```python
from build123d import *

# Parameters (mm, degrees)
EXTRUDE_1_DEPTH           = 290
HOLE_WIZARD_5_0_5_1_D     = 5
HOLE_WIZARD_5_0_5_2_D     = 5
HOLE_WIZARD_5_0_5_2_DEPTH = 20
HOLE_WIZARD_5_0_5_2_TIP   = 1.502151548


with BuildPart() as part:
    # Sketch1 → 凸台-拉伸1 (new body)
    with BuildSketch(Plane.XY):
        Polygon((-6.5, 45), (-3.2, 45), (-3.2, 43.2), (-5.1, 43.2), (-5.1, 37.2), (5.1, 37.2), (5.1, 43.2), (3.2, 43.2), (3.2, 45), (6.5, 45), (7.5, 45), (7.5, 44), (7.5, 18.2), (5, 18.2), (5, 20.2), (-0.5, 20.2), (-0.5, 18.2), (-3, 18.2), (-3, 11.8), (-0.5, 11.8), (-0.5, 9.8), (5, 9.8), (5, 11.8), (7.5, 11.8), (7.5, -11.8), (5, -11.8), (5, -9.8), (-0.5, -9.8), (-0.5, -11.8), (-3, -11.8), (-3, -18.2), (-0.5, -18.2), (-0.5, -20.2), (5, -20.2), (5, -18.2), (7.5, -18.2), (7.5, -44), (7.5, -45), (6.5, -45), (3.2, -45), (3.2, -43.2), (5.1, -43.2), (5.1, -37.2), (-5.1, -37.2), (-5.1, -43.2), (-3.2, -43.2), (-3.2, -45), (-6.496721962, -45), (-7.5, -45), (-7.5, -44), (-7.5, -33.2), (-5, -33.2), (-5, -35.2), (0.5, -35.2), (0.5, -33.2), (3, -33.2), (3, -26.8), (0.5, -26.8), (0.5, -24.8), (-5, -24.8), (-5, -26.8), (-7.5, -26.8), (-7.5, -3.2), (-5, -3.2), (-5, -5.2), (0.5, -5.2), (0.5, -3.2), (3, -3.2), (3, 3.2), (0.5, 3.2), (0.5, 5.2), (-5, 5.2), (-5, 3.2), (-7.5, 3.2), (-7.5, 26.8), (-5, 26.8), (-5, 24.8), (0.5, 24.8), (0.5, 26.8), (3, 26.8), (3, 33.2), (0.5, 33.2), (0.5, 35.2), (-5, 35.2), (-5, 33.2), (-7.5, 33.2), (-7.5, 44), (-7.5, 45), align=None)
    extrude(amount=EXTRUDE_1_DEPTH)

    # Ø5.0 (5) 直径孔1 (through all)
    with Locations(Plane(origin=(7.5, 0, 0), x_dir=(0, 0, -1), z_dir=(1, 0, 0))):
        with Locations((-268, 30)):
            Hole(HOLE_WIZARD_5_0_5_1_D / 2)

    # Ø5.0 (5) 直径孔2
    with Locations(Plane(origin=(7.5, 0, 0), x_dir=(0, 0, -1), z_dir=(1, 0, 0))):
        with Locations((-217, 30.986103622), (-181, 30.986103622), (-109, 30.986103622), (-73, 30.986103622), (-22, 30.986103622), (-268, 0), (-217, -30), (-181, -30), (-163, 0), (-127, 0), (-109, -30), (-73, -30), (-22, 0)):
            Hole(HOLE_WIZARD_5_0_5_2_D / 2, depth=HOLE_WIZARD_5_0_5_2_DEPTH)
            with Locations((0, 0, -(HOLE_WIZARD_5_0_5_2_DEPTH + HOLE_WIZARD_5_0_5_2_TIP / 2))):  # 118° drill point
                Cone(0, HOLE_WIZARD_5_0_5_2_D / 2, HOLE_WIZARD_5_0_5_2_TIP, mode=Mode.SUBTRACT)


solid = part.part
```
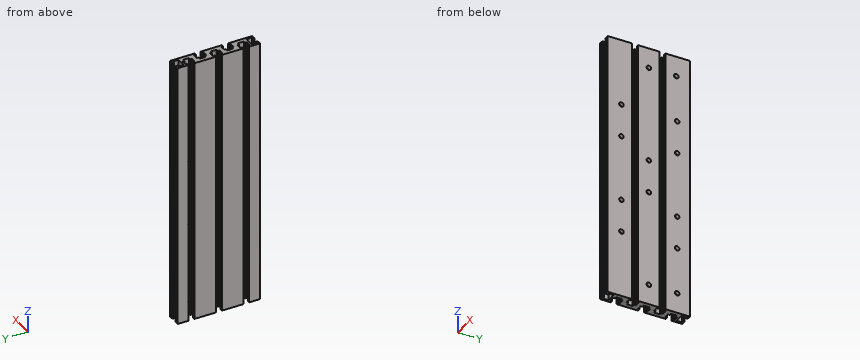
Could you check a few things on this model? Use its own coordinates, in mm. Round coordinates to 2 decimals unless told otherwise and drop trailing zeros. Order: outer loops, then holes, each group sorted by start corner. A loop starts at its lowest first (then second) coordinate and runs counter-clockwise, first axis right, second up. Notation, with made-up numbers: (30.25, -31) -> (63.25, -31) arc R16 cw to (63.25, -20) -> close; hole circle Ø7 at (58, 68.25). An arc over 180 degrees is marked (long way). One line per question, with ' | ' between items.
Q1. If we section it at C-C on y = -14.5: Write out the boundary of the cut face in (x, z).
Computed values:
outline: (-7.5, 0) -> (-3, 0) -> (-3, 290) -> (-7.5, 290) -> close
Q2. If I drill on line 1 (Y direction, x = -2.5, z = 183); line 2 (Y direction, x = 1.75, z = 107); line 3 (Y direction, x = -5.25, z = 125.5), over which ranges is the centre line in solid material (lowest first)? Write a range as from..to.
Computed values:
line 1: -37.2..-35.2, -24.8..-18.2, -11.8..-5.2, 5.2..11.8, 18.2..24.8, 35.2..37.2 | line 2: -37.2..-33.2, -26.8..-20.2, -9.8..-3.2, 3.2..9.8, 20.2..26.8, 33.2..37.2 | line 3: -45..-33.2, -26.8..-3.2, 3.2..26.8, 33.2..45
Q3. I'm going to push flat-ended pins straight in: pin 1 (3 mm diameter, centred on x = 1.5, z = 180, fed in from +Y); pin 2 (4 mm diameter, centred on y = -30, z = 73, fed in from -X); pin 3 (4 mm diameter, centred on x = -0.5, z = 163, fed in from -Y). Where does each tip first touch, or does it pass through?
Computed values:
pin 1: y = 37.2 | pin 2: through | pin 3: y = -37.2
Q4. If we section it at A-A on y = 0: Write out the boundary of the cut face in (x, z), plus the area to 4 significant figures.
Computed values:
outline: (3, 0) -> (7.5, 0) -> (7.5, 19.5) -> (3, 19.5) -> close; (3, 24.5) -> (7.5, 24.5) -> (7.5, 124.5) -> (3, 124.5) -> close; (3, 129.5) -> (7.5, 129.5) -> (7.5, 160.5) -> (3, 160.5) -> close; (3, 165.5) -> (7.5, 165.5) -> (7.5, 265.5) -> (3, 265.5) -> close; (3, 270.5) -> (7.5, 270.5) -> (7.5, 290) -> (3, 290) -> close | area: 1,215 mm²
Q5. If we section it at B-B on z = 268: Give the number of separate pieces and of enclosed holes in the cut face, plus the area to 3 significant figures.
Computed values:
separate pieces: 3 | enclosed holes: 0 | area: 714 mm²
